from build123d import *

# Parameters (mm, degrees)
F0_W     = 468.000486
F0_H     = 137.646743
F1_DEPTH = 12.954
F2_W     = 121.189991
F2_H     = 10.956902
F2_W_2   = 121.659321
F2_H_2   = 10.858484
F3_DEPTH = 11.43


with BuildPart() as f1:
    # F0 (on Top) → F1 (new body)
    with BuildSketch(Plane.XY):
        with Locations((-28.439099, 39.354104)):
            Rectangle(F0_W, F0_H)
    extrude(amount=F1_DEPTH)

    # F2 (on face) → F3 (join)
    with BuildSketch(Plane.XY.offset(12.954)):
        Polygon((123.783911, 49.460353), (123.783911, 45.553041), (-262.439342, 45.553041), (-262.439342, 41.511512), (123.529911, 41.511512), (123.51045, 37.820112), (126.581236, 37.820112), (126.581236, 41.581829), (129.575267, 41.581829), (129.575267, 37.820112), (132.569283, 37.820112), (132.569283, 41.581829), (135.793611, 41.581829), (135.793611, 37.820112), (139.017939, 37.820112), (139.017939, 41.581829), (142.395809, 41.581829), (142.395809, 37.820112), (146.157518, 37.820112), (146.157518, 41.581829), (149.535387, 41.581829), (149.535387, 37.820112), (153.066799, 37.820112), (153.066799, 41.581829), (156.060829, 41.581829), (156.060829, 37.820112), (159.054845, 37.820112), (159.054845, 41.581829), (162.279173, 41.581829), (162.279173, 37.820112), (165.503501, 37.820112), (165.503501, 41.581829), (168.881371, 41.581829), (168.881371, 37.820112), (172.64308, 37.820112), (172.64308, 41.581829), (176.02095, 41.581829), (176.02095, 37.820112), (179.806361, 37.820112), (179.806361, 41.626252), (205.451788, 41.58025), (205.451788, 45.698637), (179.806361, 45.698637), (179.806361, 49.460353), (176.27495, 49.460353), (176.27495, 45.698637), (172.89708, 45.698637), (172.89708, 49.460353), (169.135371, 49.460353), (169.135371, 45.698637), (165.757501, 45.698637), (165.757501, 49.460353), (162.533173, 49.460353), (162.533173, 45.698637), (159.308845, 45.698637), (159.308845, 49.460353), (156.314829, 49.460353), (156.314829, 45.698637), (153.320799, 45.698637), (153.320799, 49.460353), (149.789387, 49.460353), (149.789387, 45.698637), (146.411518, 45.698637), (146.411518, 49.460353), (142.649809, 49.460353), (142.649809, 45.698637), (139.271939, 45.698637), (139.271939, 49.460353), (136.047611, 49.460353), (136.047611, 45.698637), (132.823283, 45.698637), (132.823283, 49.460353), (129.829267, 49.460353), (129.829267, 45.698637), (126.835236, 45.698637), (126.835236, 49.460353), align=None)
        with Locations((-41.886206, 55.499995)):
            Rectangle(F2_W, F2_H)
        with Locations((-42.274945, 31.855833)):
            Rectangle(F2_W_2, F2_H_2)
    extrude(amount=F3_DEPTH)


solid = f1.part
Design review of the part built by this model. Coordinates are the model's own, in mm. A direction names the side the tool comes from. Coordinates: 2 decimals unless noted, no trailing zeros. Order: outer loops, then holes, each group sorted by start corner. A loop starts at its lowest first (then second) coordinate and runs counter-clockwise, first axis right, second up.
Item 1: Take a section at A-A, the plane x = -187. Write out the cut boundary in (y, z), then the cut area to 3 significant figures.
Item 2: The part is to be moulded in two halves that separate along X. For faces 1 (the flat face through (205.561, 38, 6)), 2 (the flat face through (193, 45.699, 19)), 3 (the flat face through (-262.439, 38, 7)), say which applies: pulls with the +X half, pulls with the -X half, needs draft (parallel to the pull), parting line crosses it, or undercut.
Item 3: For line 1 (Y direction, x = 10, z = 19); line 2 (Y direction, x = -183, z = 18.25); line 3 (Z direction, x = -22, y = 91.5), list the stretches that pass through material, from the lowest coordinate up.
Item 4: For pin 1 Ø3 at (y, z) = (50, 15) entering from +X; pin 2 Ø12.5 at (x, z) = (-46, 20) entering from -Y; pin 3 Ø3 at (x, z) = (-156, 14.5) entering from -Y, all flat-tipped, find the tip position at first contact; note any pin that passes through.
Item 5: For faces 4 (the flat face through (-43, 26.427, 19)), 5 (the flat face through (-103.105, 32, 19)), 6 (the flat face through (-43, 37.285, 19)), 7 (the flat face through (18.555, 32, 19)), 8 (the flat face through (18.709, 55, 19)), list the 3-axis set-ups (+Z, -Z, +X, -X, +Y, -Y) from which the entire face can be reached by the end or side of a thin tool; tool diameter is ignored.
Item 6: Take a section at C-C, the plane z = 18.75. Count the separate pieces of the cut face and the enclosed holes in it, then the cut area to 3 significant figures.
Item 7: Take a section at D-D, the plane x = -12. Write out the cut boundary in (y, z).
Item 8: Take a section at B-B, the plane y = 55.5. Write out the cut boundary in (x, z).
The answers:
1. outline: (-29.47, 0) - (108.18, 0) - (108.18, 12.95) - (45.55, 12.95) - (45.55, 24.38) - (41.51, 24.38) - (41.51, 12.95) - (-29.47, 12.95) - close
1. area: 1,830 mm2
2. face 1: pulls with the +X half
2. face 2: needs draft
2. face 3: pulls with the -X half
3. line 1: y = 26.43 to 37.29, 41.51 to 45.55, 50.02 to 60.98
3. line 2: y = 41.51 to 45.55
3. line 3: z = 0 to 12.95
4. pin 1: stops at x = 179.81
4. pin 2: stops at y = 26.43
4. pin 3: stops at y = 41.51
5. face 4: +Z, +X, -X, -Y
5. face 5: +Z, -X, -Y
5. face 6: +Z, +X, -X
5. face 7: +Z, +X, -Y
5. face 8: +Z, +X, +Y
6. separate pieces: 3
6. enclosed holes: 0
6. area: 4,770 mm2
7. outline: (-29.47, 0) - (108.18, 0) - (108.18, 12.95) - (60.98, 12.95) - (60.98, 24.38) - (50.02, 24.38) - (50.02, 12.95) - (45.55, 12.95) - (45.55, 24.38) - (41.51, 24.38) - (41.51, 12.95) - (37.29, 12.95) - (37.29, 24.38) - (26.43, 24.38) - (26.43, 12.95) - (-29.47, 12.95) - close
8. outline: (-262.44, 0) - (205.56, 0) - (205.56, 12.95) - (18.71, 12.95) - (18.71, 24.38) - (-102.48, 24.38) - (-102.48, 12.95) - (-262.44, 12.95) - close
